Drawing for the job (mm, zero at the part's lowest x, y, z). A direction names the side the tool comes from. Round coordinates to 2 decimals unless told otherwise and drop trailing zeros. Order: outer loops, then holes, each group sorted by start corner. A loop starts at its lowest first (then second) coordinate and runs counter-clockwise, first axis right, second up. Notation, with made-up numbers: (68, 21.5) -> (118, 21.5) arc R10 ccw to (118, 39.5) -> close; hole circle Ø3 at (-19, 28). An arc over 180 degrees is marked (long way). Use CSV: the item, a comma, the result in double quotes.
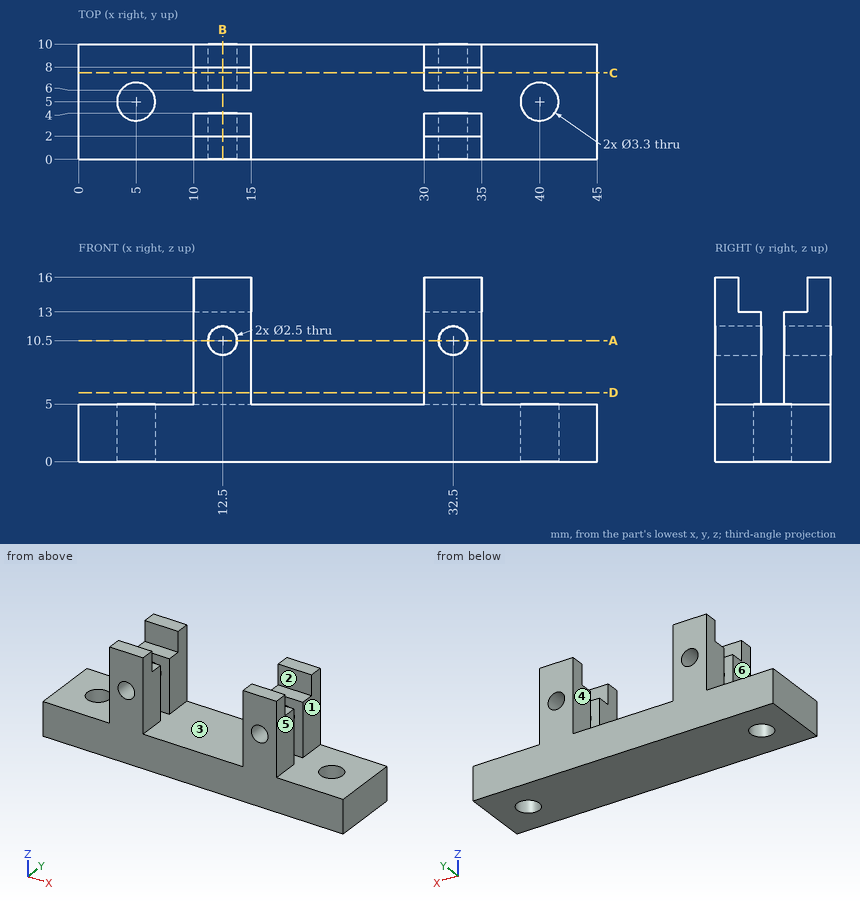
Q1. Pin check, flat tips, straight feed: pin 1 (6 mm diameter, centred on x = 25.5, z = 9, fed in from -Y); pin 2 (1 mm diameter, centred on y = 6, z = 10, fed in from +X); pin 3 (0.6 mm diameter, centred on x = 31.5, y = 6.5, fed in from +Z); pin 4 (4.5 mm diameter, centred on y = 2, z = 8, fed in from -X). Stop position of each tip, or through.
From the geometry:
pin 1,"passes through"
pin 2,"stops at x = 35"
pin 3,"stops at z = 13"
pin 4,"stops at x = 10"
Q2. Cut at D-D (z = 6). Give the cut face in (x, y).
From the geometry:
outline,"(10, 0) -> (15, 0) -> (15, 4) -> (10, 4) -> close; (10, 6) -> (15, 6) -> (15, 10) -> (10, 10) -> close; (30, 0) -> (35, 0) -> (35, 4) -> (30, 4) -> close; (30, 6) -> (35, 6) -> (35, 10) -> (30, 10) -> close"
Q3. Which spindle directions (+Z, -Z, +X, -X, +Y, -Y) get a long thin tool onto all of the face, cutting with end or side? Do the marked faces 4, 5 and 6. Say none if no direction does.
From the geometry:
face 4,"+Z, +Y, -Y"
face 5,"+Z, +X, +Y, -Y"
face 6,"+Z, -X, +Y, -Y"
Q4. Probe line 1 along X through (y, z) = (1.7, 10.5); line 2 along Y through (x, z) = (32, 6.5); line 3 along Z through (x, y) = (12.5, 3.15). List the from-to ranges inside material, lowest first.
From the geometry:
line 1,"x = 10 to 11.25, 13.75 to 15, 30 to 31.25, 33.75 to 35"
line 2,"y = 0 to 4, 6 to 10"
line 3,"z = 0 to 9.25, 11.75 to 13"
Q5. Mould opens along X. For the marked faces 1, 2 and 3 say: +X half, -X half, draft (parallel to the pull), parting line (faces both ways), or undercut.
From the geometry:
face 1,"+X half"
face 2,"draft"
face 3,"undercut"
Q6. Cut at B-B (x = 12.5). Give the cut face in (y, z), plus the area to 3 significant figures.
From the geometry:
outline,"(0, 0) -> (10, 0) -> (10, 9.25) -> (6, 9.25) -> (6, 5) -> (4, 5) -> (4, 9.25) -> (0, 9.25) -> close; (0, 11.75) -> (4, 11.75) -> (4, 13) -> (2, 13) -> (2, 16) -> (0, 16) -> close; (6, 11.75) -> (10, 11.75) -> (10, 16) -> (8, 16) -> (8, 13) -> (6, 13) -> close"
area,"106 mm²"
Q7. Cut at C-C (y = 7.5). Give the cut face in (x, z).
From the geometry:
outline,"(0, 0) -> (45, 0) -> (45, 5) -> (35, 5) -> (35, 13) -> (30, 13) -> (30, 5) -> (15, 5) -> (15, 13) -> (10, 13) -> (10, 5) -> (0, 5) -> close; hole circle Ø2.5 at (12.5, 10.5); hole circle Ø2.5 at (32.5, 10.5)"
Q8. Cut at A-A (z = 10.5). State how many separate pieces and enclosed holes the cut face has, plus the area to 3 significant figures.
From the geometry:
separate pieces,"8"
enclosed holes,"0"
area,"40.0 mm²"
